Here's how the part is built. I have some questions about the finished solid (model axes, mm). Face numbers are marked on the shaded views. A direction names the side the tool comes from. Coordinates: 2 decimals unless noted, no trailing zeros. Order: outer loops, then holes, each group sorted by start corner. A loop starts at its lowest first (then second) coordinate and runs counter-clockwise, first axis right, second up. Notation, with made-up numbers: (36.5, -32) - (77.5, -32) arc R16 ccw to (77.5, -20) - close; hole circle Ø5 at (-16.5, 84). An arc over 180 degrees is marked (long way). Answer as CSV lines item,"result". Start each with the question number.
Item 1: Imagine slicing it at A-A on z = 23.5. List the corners of the cut face in (x, y) for me, and give its area (3 significant figures).
Item 2: I'm going to push flat-ended pins straight in: pin 1 (1.5 mm diameter, centred on x = -7.5, z = 15, fed in from +Y); pin 2 (1.5 mm diameter, centred on x = -5, z = 22, fed in from +Y); pin 3 (2 mm diameter, centred on x = 11.5, z = 4, fed in from -Y). Where does each tip first touch, or does it pass through?
Item 3: Imagine slicing it at C-C on z = 3.5. List the corners of the cut face in (x, y) for me, and give its area (3 significant figures).
Item 4: Imagine slicing it at B-B on x = 0. List the corners of the cut face in (y, z) for me, and give its area (3 significant figures).
Item 5: I need wall thicknesses on line 1 (Y direction, x = 0, z = 8.35); line 2 (Y direction, x = 0, z = 5.1); line 3 (X direction, y = -2.5, z = 20.25). Which ranges of each line are inside material? Lowest first, please.
Item 6: We'd pull the mould along X, two halves only. Please class the marked faces 3, 4, 5 and 6: pulls with the +X half, pulls with the -X half, needs draft (parallel to the pull), parting line crosses it, or undercut.
Item 7: On a 3-axis mill with a long thin cutter (end or side, diameter ignored), from which of +Z, -Z, +X, -X, +Y, -Y can I reach the whole of each face in a straight line? I mean the marked faces 1 and 2. Say none if no direction works.
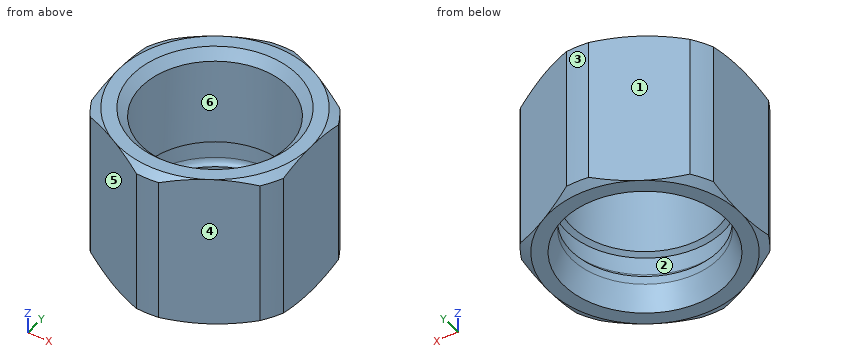
from build123d import *

# Parameters (mm, degrees)
SKETCH_1_R          = 12.25
EXTRUDE_1_DEPTH     = 26
SKETCH_7_OUTSIDE_W  = 45.074
SKETCH_7_OUTSIDE_H  = 50.024
SKETCH_7_OUTSIDE_R  = 17.5
CUT_EXTRUDE_2_DEPTH = 36.68379651
CHAMFER_1_SIZE      = 1.5


with BuildPart() as part:
    # Эскиз1 → Бобышка-Вытянуть1 (new body)
    with BuildSketch(Plane.XY):
        Polygon((0, 18.475208614), (-16, 9.237604307), (-16, -9.237604307), (0, -18.475208614), (16, -9.237604307), (16, 9.237604307), align=None)
        with Locations(Location((0, 0, 0), (0, 0, 180))):
            Circle(SKETCH_1_R, mode=Mode.SUBTRACT)
    extrude(amount=EXTRUDE_1_DEPTH)

    # Эскиз2 → Вырез-Повернуть1 (revolve, cut)
    with BuildSketch(Plane(origin=(0, 0, 0), x_dir=(0, 0, -1), z_dir=(1, 0, 0))):
        Polygon((0, 19.828002546), (-2.210098301, 19.828002546), (0, 16), align=None)
        Polygon((-23.789901699, 19.828002546), (-26, 16), (-26, 19.828002546), align=None)
    revolve(axis=Axis((0, 0, 0), (0, 0, 1)), mode=Mode.SUBTRACT)

    # Эскиз7 outside → Вырез-Вытянуть2 (cut, through all)
    with BuildSketch(Plane.XY.offset(26)):
        Rectangle(SKETCH_7_OUTSIDE_W, SKETCH_7_OUTSIDE_H)
        Circle(SKETCH_7_OUTSIDE_R, mode=Mode.SUBTRACT)
    extrude(amount=-CUT_EXTRUDE_2_DEPTH, mode=Mode.SUBTRACT)

    # Эскиз3 → Вырез-Повернуть2 (revolve, cut)
    with BuildSketch(Plane(origin=(0, 0, 0), x_dir=(0, 0, -1), z_dir=(1, 0, 0)), mode=Mode.PRIVATE) as cut_revolve_2_sk:
        with BuildLine():
            Line((-9.5, 13.1), (-11.145448267, 10.25))
            Line((-11.145448267, 10.25), (0.758835928, 10.25))
            Line((0.758835928, 10.25), (0.758835928, 13.832407636))
            Line((0.758835928, 13.832407636), (-4.111314003, 12.25))
            Line((-4.111314003, 12.25), (-5.511314003, 12.25))
            ThreePointArc((-5.511314003, 12.25), (-5.848079759, 12.858287544), (-6.5, 13.1))
            Line((-6.5, 13.1), (-9.5, 13.1))
        make_face()
    revolve(cut_revolve_2_sk.sketch.rotate(Axis((0, 0, 0), (0, 0, 1)), 90), axis=Axis((0, 0, 0), (0, 0, 1)), mode=Mode.SUBTRACT)

    # Фаска1
    chamfer_1_edges = [part.edges().sort_by_distance(p)[0] for p in [
        (12.25, 0, 26),
    ]]
    chamfer(chamfer_1_edges, length=CHAMFER_1_SIZE)


solid = part.part
Responses:
1,outline,"(-16, -7.09) arc R17.5 ccw to (-14.14, -10.31) - (-1.86, -17.4) arc R17.5 ccw to (1.86, -17.4) - (14.14, -10.31) arc R17.5 ccw to (16, -7.09) - (16, 7.09) arc R17.5 ccw to (14.14, 10.31) - (1.86, 17.4) arc R17.5 ccw to (-1.86, 17.4) - (-14.14, 10.31) arc R17.5 ccw to (-16, 7.09) - close; hole circle Ø24.5 at (0, 0)"
1,area,"405 mm^2"
2,pin 1,"stops at y = 14.58"
2,pin 2,"stops at y = 16.02"
2,pin 3,"stops at y = -12.41"
3,outline,"(-16, -7.09) arc R17.5 ccw to (-14.14, -10.31) - (-1.86, -17.4) arc R17.5 ccw to (1.86, -17.4) - (14.14, -10.31) arc R17.5 ccw to (16, -7.09) - (16, 7.09) arc R17.5 ccw to (14.14, 10.31) - (1.86, 17.4) arc R17.5 ccw to (-1.86, 17.4) - (-14.14, 10.31) arc R17.5 ccw to (-16, 7.09) - close; hole circle Ø24.9 at (0, 0)"
3,area,"389 mm^2"
4,outline,"(-17.5, 0.87) - (-16, 0) - (-13.59, 0) - (-12.25, 4.11) - (-12.25, 5.51) arc R1 cw to (-13.1, 6.5) - (-13.1, 9.5) - (-12.25, 9.99) - (-12.25, 24.5) - (-13.75, 26) - (-16, 26) - (-17.5, 25.13) - close; (12.25, 4.11) - (13.59, 0) - (16, 0) - (17.5, 0.87) - (17.5, 25.13) - (16, 26) - (13.75, 26) - (12.25, 24.5) - (12.25, 9.99) - (13.1, 9.5) - (13.1, 6.5) arc R1 cw to (12.25, 5.51) - close"
4,area,"256 mm^2"
5,line 1,"y = -17.5 to -13.1, 13.1 to 17.5"
5,line 2,"y = -17.5 to -12.25, 12.25 to 17.5"
5,line 3,"x = -16 to -11.99, 11.99 to 16"
6,face 3,"parting line crosses it"
6,face 4,"pulls with the +X half"
6,face 5,"pulls with the -X half"
6,face 6,"undercut"
7,face 1,"+Z, -Z, -X, +Y"
7,face 2,"none"
